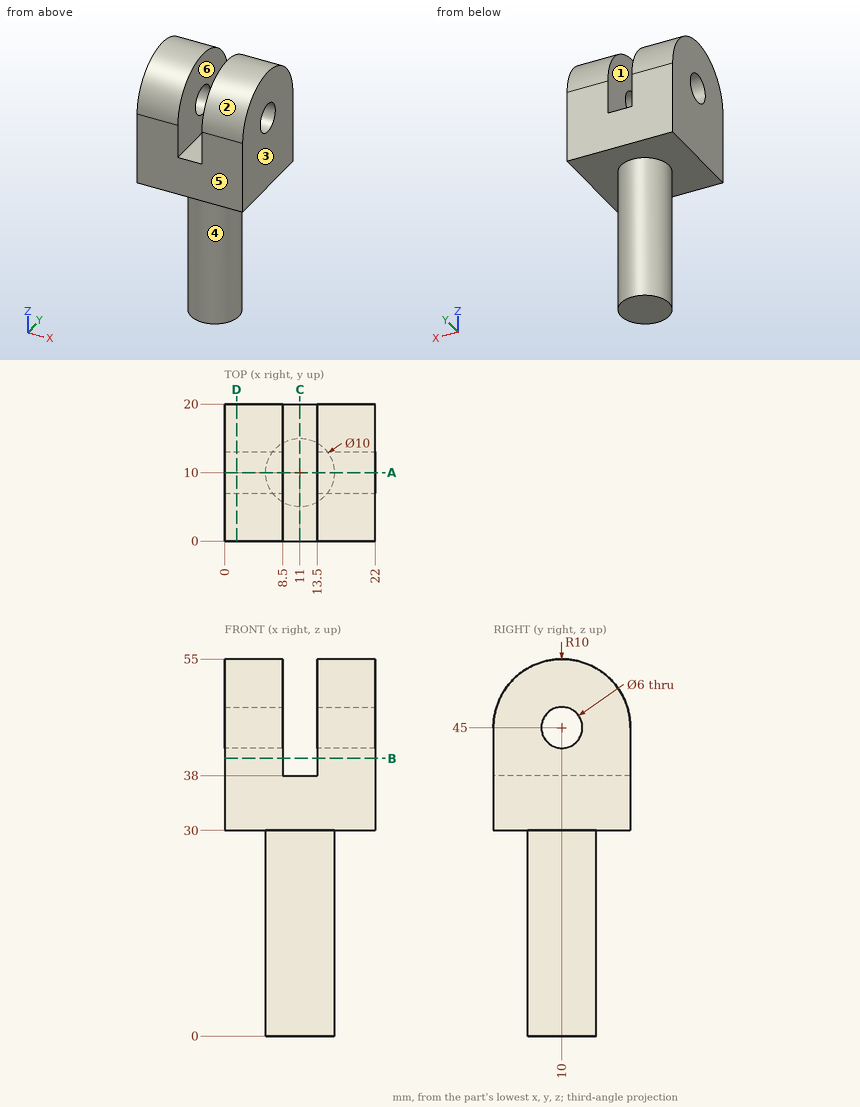
Could you check a few things on this drawing? It's one solid part, dimensions in mm from its lowest x, y, z. A direction names the side the tool comes from. Coordinates: 2 decimals unless noted, no trailing zeros. Order: outer loops, then holes, each group sorted by start corner. A loop starts at its lowest first (then second) coordinate and runs counter-clockwise, first axis right, second up.
1. If we section it at D-D (x = 1.75): Please give me the cut outline in (y, z).
2. I need wall thicknesses on line 1 (Y direction, x = 2, z = 45); line 2 (X direction, y = 14, z = 49); line 3 (X direction, y = 10, z = 3). Which ranges of each line are inside material? Lowest first, please.
3. For the marked faces 4, 5 and 6, which set-ups out of +Z, -Z, +X, -X, +Y, -Y let a thin tool reach every point of the face, with its end or its side?
4. If we section it at C-C (x = 11): Please give me the cut outline in (y, z), then the cut area to 3 significant figures.
5. I'm going to push flat-ended pins straight in: pin 1 (1.5 mm diameter, centred on x = 10.5, y = 14.5, fed in from +Z); pin 2 (6 mm diameter, centred on x = 15, z = 21.5, fed in from -Y); pin 3 (3 mm diameter, centred on y = 5.5, z = 12, fed in from -X). Where does each tip first touch, or does it pass through?
6. Thinking about a two-plate mould opening in X: for the marked faces 1, 2 and 3, which applies, +X half, -X half, draft (parallel to the pull), parting line (faces both ways), or undercut?
7. If we section it at B-B (z = 40.5): Please give me the cut outline in (x, y), then the cut area to 3 significant figures.
8. If we section it at A-A (y = 10): Please give me the cut outline in (x, z).
Entries:
1. outline: (0, 30) - (20, 30) - (20, 45) arc R10 ccw to (0, 45) - close; hole circle Ø6 at (10, 45)
2. line 1: y = 0 to 7, 13 to 20
2. line 2: x = 0 to 8.5, 13.5 to 22
2. line 3: x = 6 to 16
3. face 4: -Z
3. face 5: +Z, -Z, +X, -X, -Y
3. face 6: +Z, +Y, -Y
4. outline: (0, 30) - (5, 30) - (5, 0) - (15, 0) - (15, 30) - (20, 30) - (20, 38) - (0, 38) - close
4. area: 460 mm2
5. pin 1: stops at z = 38
5. pin 2: stops at y = 5.1
5. pin 3: stops at x = 7
6. face 1: undercut
6. face 2: draft
6. face 3: +X half
7. outline: (0, 0) - (8.5, 0) - (8.5, 20) - (0, 20) - close; (13.5, 0) - (22, 0) - (22, 20) - (13.5, 20) - close
7. area: 340 mm2
8. outline: (0, 30) - (6, 30) - (6, 0) - (16, 0) - (16, 30) - (22, 30) - (22, 42) - (13.5, 42) - (13.5, 38) - (8.5, 38) - (8.5, 42) - (0, 42) - close; (0, 48) - (8.5, 48) - (8.5, 55) - (0, 55) - close; (13.5, 48) - (22, 48) - (22, 55) - (13.5, 55) - close
